from build123d import *

# Parameters (mm, degrees)
BOSS_EXTRUDE2_DEPTH = 1
BOSS_EXTRUDE3_DEPTH = 6
SKETCH3_R           = 1.5
CUT_EXTRUDE1_DEPTH  = 6
FILLET1_R           = 2
SKETCH4_W           = 1
SKETCH4_H           = 4
BOSS_EXTRUDE4_DEPTH = 6.5


with BuildPart() as part:
    # Sketch1 → Boss-Extrude2 (new body)
    with BuildSketch(Plane.XY):
        with BuildLine():
            Line((7.5, 0), (7.5, -6.5))
            Line((7.5, -6.5), (6.5, -6.5))
            Line((6.5, -6.5), (6.5, 0))
            ThreePointArc((6.5, 0), (0, 6.5), (-6.5, 0))
            Line((-6.5, 0), (-6.5, -6.5))
            Line((-6.5, -6.5), (-7.5, -6.5))
            Line((-7.5, -6.5), (-7.5, 0))
            ThreePointArc((-7.5, 0), (0, 7.5), (7.5, 0))
        make_face()
    boss_extrude2 = extrude(amount=BOSS_EXTRUDE2_DEPTH)

    # Sketch1<4> → Boss-Extrude3 (add)
    with BuildSketch(Plane.XY):
        with BuildLine():
            Line((-7.5, -6.5), (-6.5, -6.5))
            ThreePointArc((-6.5, -6.5), (-7.085786438, -7.914213562), (-8.5, -8.5))
            Line((-8.5, -8.5), (-15, -8.5))
            Line((-15, -8.5), (-15, -7.5))
            Line((-15, -7.5), (-8.5, -7.5))
            ThreePointArc((-8.5, -7.5), (-7.792893219, -7.207106781), (-7.5, -6.5))
        make_face()
        with BuildLine():
            Line((6.5, -6.5), (7.5, -6.5))
            ThreePointArc((7.5, -6.5), (7.792893219, -7.207106781), (8.5, -7.5))
            Line((8.5, -7.5), (15, -7.5))
            Line((15, -7.5), (15, -8.5))
            Line((15, -8.5), (8.5, -8.5))
            ThreePointArc((8.5, -8.5), (7.085786438, -7.914213562), (6.5, -6.5))
        make_face()
    extrude(amount=BOSS_EXTRUDE3_DEPTH)

    # Mirror1: Boss-Extrude2 across plane
    add(boss_extrude2.mirror(Plane.XY.offset(3)))

    # Sketch3 → Cut-Extrude1 (cut)
    with BuildSketch(Plane(origin=(0, -7.5, 0), x_dir=(1, 0, 0), z_dir=(0, 1, 0))):
        with Locations(Location((-11.75, -3, 0), (0, 0, 180))):
            Circle(SKETCH3_R)
    cut_extrude1 = extrude(amount=-CUT_EXTRUDE1_DEPTH, mode=Mode.SUBTRACT)

    # Mirror2: Cut-Extrude1 across plane
    add(cut_extrude1.mirror(Plane.ZY), mode=Mode.SUBTRACT)

    # Fillet1
    fillet1_edges = [part.edges().sort_by_distance(p)[0] for p in [
        (-15, -8, 0),
        (-15, -8, 6),
        (15, -8, 6),
        (15, -8, 0),
    ]]
    fillet(fillet1_edges, radius=FILLET1_R)

    # Sketch4 → Boss-Extrude4 (add)
    with BuildSketch(Plane(origin=(0, -6.5, 0), x_dir=(1, 0, 0), z_dir=(0, 1, 0))):
        with Locations((7, -3)):
            Rectangle(SKETCH4_W, SKETCH4_H)
        with Locations((-7, -3)):
            Rectangle(SKETCH4_W, SKETCH4_H)
    extrude(amount=BOSS_EXTRUDE4_DEPTH)


solid = part.part
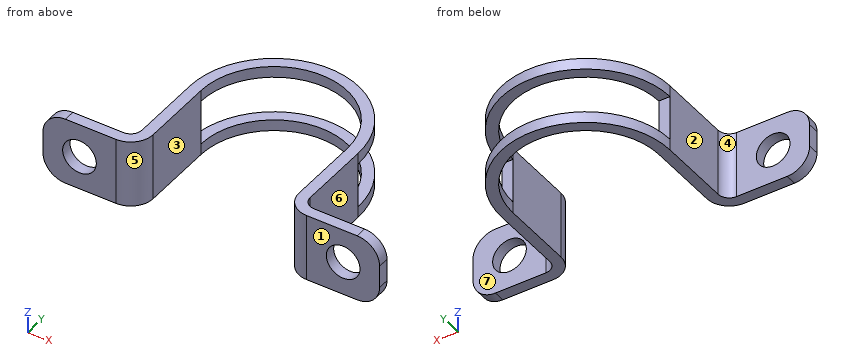
Check sheet for the modelled part. Datum: model origin and axes. Units: mm. Face numbers are marked on the shaded views. A direction names the side the tool comes from. Round coordinates to 2 decimals unless told otherwise and drop trailing zeros. Loops run counter-clockwise (first coordinate to the right, second up) from the corner with the lowest first, then second, coordinate; pieces in that order, holes last. Notation, with made-up numbers: (83.25, 23) -> (142.25, 23) arc R17 ccw to (142.25, 51) -> close; hole circle Ø7 at (63.5, -12.75). An arc over 180 degrees is marked (long way). Put each result on its own line as item: value. Start each with the question number.
1. Draft check along X on the marked faces 4, 5, 6 and 7. Enter one of: +X half, -X half, draft (parallel to the pull), parting line (faces both ways), or undercut.
2. Access from +Z, -Z, +X, -X, +Y, -Y to the whole of each face (thin tool, end or side, straight path). Record for the marked faces 1, 2 and 3.
3. Section check B-B (z = 3). Enter the section's corners in (x, y), plus the area to 3 significant figures.
4. Section check A-A (x = 0). Enter the section's corners in (y, z).
5. Section check D-D (y = -3.5). Enter the section's corners in (x, z).
6. Scan lines: probe 1 along X at (y, z) = (-3.5, 4.7); probe 2 along Z at (x, y) = (-7.25, 1); probe 3 along Z at (x, y) = (-11.75, -8). Record each from-to range of solid material in increasing order.
7. Section check C-C (y = 0.5). Enter the section's corners in (x, z), plus the area to 3 significant figures.
8. Gauge pin test, flat ends, axial feed: pin 1 (3 mm diameter, centred on y = -2.5, z = 2, fed in from -X); pin 2 (1.8 mm diameter, centred on x = -11.75, z = 3, fed in from +Y); pin 3 (1.8 mm diameter, centred on y = -3, z = 2, fed in from +X); pin 4 (0.8 mm diameter, centred on x = 7, z = 3, fed in from +Y). Record the tip position at first contact, or that the pin passes through.
Findings:
1. face 4: -X half
1. face 5: undercut
1. face 6: +X half
1. face 7: draft
2. face 1: +Z, -Z, +X, -X, -Y
2. face 2: +Z, -Z, -X, +Y
2. face 3: +Z, -Z, -Y
3. outline: (-15, -8.5) -> (-13.25, -8.5) -> (-13.25, -7.5) -> (-15, -7.5) -> close; (-10.25, -8.5) -> (-8.5, -8.5) arc R2 ccw to (-6.5, -6.5) -> (-6.5, 0) -> (-7.5, 0) -> (-7.5, -6.5) arc R1 cw to (-8.5, -7.5) -> (-10.25, -7.5) -> close; (6.5, -6.5) arc R2 ccw to (8.5, -8.5) -> (10.25, -8.5) -> (10.25, -7.5) -> (8.5, -7.5) arc R1 cw to (7.5, -6.5) -> (7.5, 0) -> (6.5, 0) -> close; (13.25, -8.5) -> (15, -8.5) -> (15, -7.5) -> (13.25, -7.5) -> close
3. area: 24.7 mm^2
4. outline: (6.5, 0) -> (7.5, 0) -> (7.5, 1) -> (6.5, 1) -> close; (6.5, 5) -> (7.5, 5) -> (7.5, 6) -> (6.5, 6) -> close
5. outline: (-7.5, 0) -> (-6.5, 0) -> (-6.5, 6) -> (-7.5, 6) -> close; (6.5, 0) -> (7.5, 0) -> (7.5, 6) -> (6.5, 6) -> close
6. probe 1: x = -7.5 to -6.5, 6.5 to 7.5
6. probe 2: z = 0 to 1, 5 to 6
6. probe 3: z = 0 to 1.5, 4.5 to 6
7. outline: (-7.48, 0) -> (-6.48, 0) -> (-6.48, 1) -> (-7.48, 1) -> close; (-7.48, 5) -> (-6.48, 5) -> (-6.48, 6) -> (-7.48, 6) -> close; (6.48, 0) -> (7.48, 0) -> (7.48, 1) -> (6.48, 1) -> close; (6.48, 5) -> (7.48, 5) -> (7.48, 6) -> (6.48, 6) -> close
7. area: 4.01 mm^2
8. pin 1: stops at x = -7.5
8. pin 2: passes through
8. pin 3: stops at x = 7.5
8. pin 4: stops at y = 0
